Can you work these out from the model? Positions are in its coordinate system, mm. Face numbers are marked on the shaded views. A direction names the side the tool comes from. Coordinates: 2 decimals unless noted, no trailing zeros. Loops run counter-clockwise (first coordinate to the right, second up) from the corner with the lowest first, then second, coordinate; pieces in that order, holes last. Notation, with made-up numbers: (51, -24.5) -> (84, -24.5) arc R28 ccw to (84, 10.5) -> close; hole circle Ø3 at (82.25, -38.5). An arc over 180 degrees is marked (long way). Put each result on its own line as item: value. Start each with the question number.
Item 1: For the marked faces 1 and 2, which set-ups out of +Z, -Z, +X, -X, +Y, -Y let a thin tool reach every point of the face, with its end or its side?
Item 2: If we section it at A-A on x = 0: Please give me the cut outline in (y, z), plus the area to 3 significant figures.
Item 3: If we section it at C-C on z = -248: Please give me the cut outline in (x, y) (1 decimal), plus the area to 3 significant figures.
Item 4: Please list where these lines run through material, in increasing order: L1, parallel to Y at x = 0, z = -172; L2, parallel to Y at x = -1, z = -239. Write a range as from..to.
Item 5: Will these pins go through, and if not, where does the flat tip stop? P1, Ø4, axis at y = -376.5, z = 62, coming from the -X side; P2, Ø5, axis at x = -9.5, z = -73, coming from the +Y side; P3, Ø10, axis at x = -1.5, z = -64, coming from the -Y side.
```python
from build123d import *

# Parameters (mm, degrees)
SKETCH3_R           = 12.7
SKETCH3_R_2         = 4.7625
SKETCH4_R           = 12.7
SKETCH4_R_2         = 4.7625
BOSS_EXTRUDE3_DEPTH = 609.6
SKETCH5_R           = 12.7
SKETCH5_R_2         = 4.7625
BOSS_EXTRUDE4_DEPTH = 330.2
SKETCH6_W           = 12.7
SKETCH6_H           = 609.6
CUT_EXTRUDE1_DEPTH  = 6.35


with BuildPart() as part:
    # Sweep1: sweep along a path in Sketch2
    with BuildLine(Plane(origin=(0, 0, 0), x_dir=(0, 0, -1), z_dir=(1, 0, 0))) as sweep1_path:
        ThreePointArc((-64.833774642, 0), (-45.844401699, 45.844401699), (0, 64.833774642))
    # Sketch3 → Sweep1 (sweep)
    with BuildSketch(Plane(origin=(0, 0, 0), x_dir=(1, 0, 0), z_dir=(0, 1, 0))):
        with Locations((0, -64.833774642)):
            Circle(SKETCH3_R)
        with Locations((0, -64.833774642)):
            Circle(SKETCH3_R_2, mode=Mode.SUBTRACT)
    sweep(path=sweep1_path.line)

    # Sketch4 → Boss-Extrude3 (add)
    with BuildSketch(Plane(origin=(0, 0, 0), x_dir=(-1, 0, 0), z_dir=(0, -1, 0))):
        with Locations((0, -64.833774642)):
            Circle(SKETCH4_R)
        with Locations((0, -64.833774642)):
            Circle(SKETCH4_R_2, mode=Mode.SUBTRACT)
    extrude(amount=BOSS_EXTRUDE3_DEPTH)

    # Sketch5 → Boss-Extrude4 (add)
    with BuildSketch(Plane(origin=(0, 0, 0), x_dir=(-1, 0, 0), z_dir=(0, 0, -1))):
        with Locations((0, 64.833774642)):
            Circle(SKETCH5_R)
        with Locations((0, 64.833774642)):
            Circle(SKETCH5_R_2, mode=Mode.SUBTRACT)
    extrude(amount=BOSS_EXTRUDE4_DEPTH)

    # Sketch6 → Cut-Extrude1 (cut)
    with BuildSketch(Plane.ZY.offset(12.7)):
        with Locations((63.5, -304.8)):
            Rectangle(SKETCH6_W, SKETCH6_H)
    extrude(amount=-CUT_EXTRUDE1_DEPTH, mode=Mode.SUBTRACT)


solid = part.part
```
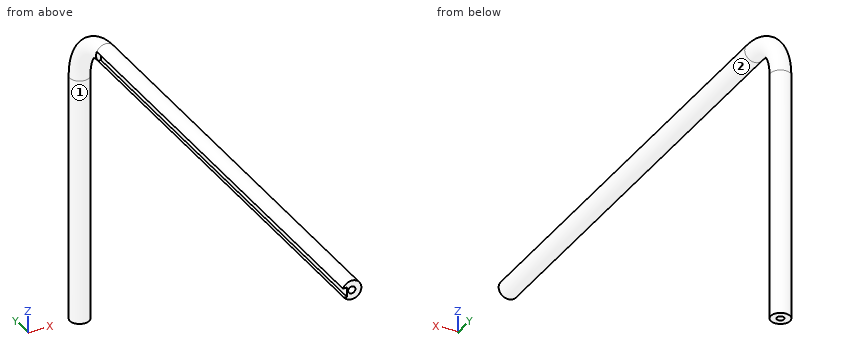
Solutions:
1. face 1: -Z
1. face 2: -Y
2. outline: (-609.6, 52.13) -> (0, 52.13) arc R52.13 cw to (52.13, 0) -> (52.13, -330.2) -> (60.07, -330.2) -> (60.07, 0) arc R60.07 ccw to (0, 60.07) -> (-609.6, 60.07) -> close; (-609.6, 69.6) -> (0, 69.6) arc R69.6 cw to (69.6, 0) -> (69.6, -330.2) -> (77.53, -330.2) -> (77.53, 0) arc R77.53 ccw to (0, 77.53) -> (-609.6, 77.53) -> close
2. area: 16,500 mm^2
3. outline: circle Ø25.4 at (0, 64.8); hole circle Ø9.5 at (0, 64.8)
3. area: 435 mm^2
4. L1: 52.13..60.07, 69.6..77.53
4. L2: 52.17..60.18, 69.49..77.49
5. P1: x = -6.35
5. P2: y = 75.43
5. P3: y = 52.13
